Source: CAD feature listing. Evaluate the final solid. Frame: model axes, mm. A direction names the side the tool comes from. Give positions to 0.01 mm unless a question says otherwise; leave off trailing zeros. Order: outer loops, then holes, each group sorted by start corner. A loop starts at its lowest first (then second) coordinate and runs counter-clockwise, first axis right, second up. Notation, with made-up numbers: (58.5, 11.5) - (96.5, 11.5) arc R15 cw to (96.5, 21.5) - close; hole circle Ø6 at (28.5, -14.75). An arc over 180 degrees is marked (long way). Use CSV: the item, a comma, the result in double quotes.
```python
from build123d import *

# Parameters (mm, degrees)
F0_W      = 38.1
F0_H      = 19.05
F1_DEPTH  = 50.8
F3_D      = 9.8044
F4_W      = 50.8
F4_H      = 19.05
F4_H_2    = 38.1
F5_DEPTH  = 12.7
F7_W      = 40.64
F7_H      = 43.18
F8_DEPTH  = 69.85
F9_W      = 40.64
F9_H      = 43.18
F10_DEPTH = 6.35
F12_DEPTH = 9.525
F14_D     = 3.4544
F14_DEPTH = 12.7
F14_TIP   = 1.0378064612
F15_R     = 12.7
F16_R     = 12.7
F17_R     = 4.7625
F19_DEPTH = 25.4


with BuildPart() as f1:
    # F0 (on Right) → F1 (new body)
    with BuildSketch(Plane.YZ):
        Polygon((0, 63.5), (0, 0), (19.05, 0), (57.15, 0), (76.2, 0), (76.2, 63.5), align=None)
        with Locations((38.1, -9.525)):
            Rectangle(F0_W, F0_H)
    extrude(amount=F1_DEPTH)

    # F3 (through all)
    with Locations(Plane(origin=(0, 0, 0), x_dir=(0, -1, 0), z_dir=(-1, 0, 0))):
        with Locations((-38.1, 31.75)):
            Hole(F3_D / 2)

    # F4 (on face) → F5 (join)
    with BuildSketch(Plane(origin=(0, 0, -19.05), x_dir=(1, 0, 0), z_dir=(0, 0, -1))):
        with Locations((25.4, -9.525)):
            Rectangle(F4_W, F4_H)
        with Locations((25.4, -66.675)):
            Rectangle(F4_W, F4_H)
        with Locations((25.4, -38.1)):
            Rectangle(F4_W, F4_H_2)
    extrude(amount=F5_DEPTH)

    # F7 (on face) → F8 (cut)
    with BuildSketch(Plane.XZ):
        with Locations((30.48, 31.75)):
            Rectangle(F7_W, F7_H)
    extrude(amount=-F8_DEPTH, mode=Mode.SUBTRACT)

    # F9 (on face) → F10 (cut)
    with BuildSketch(Plane.XZ):
        with Locations((30.48, 31.75)):
            Rectangle(F9_W, F9_H)
        Polygon((50.8, 53.34), (50.8, 56.515), (6.985, 56.515), (6.985, 6.985), (50.8, 6.985), (50.8, 10.16), (10.16, 10.16), (10.16, 53.34), align=None)
    extrude(amount=-F10_DEPTH, mode=Mode.SUBTRACT)

    # F11 (on face) → F12 (cut)
    with BuildSketch(Plane.YZ.offset(50.8)):
        Polygon((19.05, -19.05), (0, -19.05), (0, -31.75), (76.2, -31.75), (76.2, -19.05), (57.15, -19.05), align=None)
    extrude(amount=-F12_DEPTH, mode=Mode.SUBTRACT)

    # F14
    with Locations(Plane.YZ.offset(50.8)):
        with Locations((12.7, 58.42), (63.5, 58.42), (12.7, 5.08), (63.5, 5.08)):
            Hole(F14_D / 2, depth=F14_DEPTH)
            with Locations((0, 0, -(F14_DEPTH + F14_TIP / 2))):  # 118° drill point
                Cone(0, F14_D / 2, F14_TIP, mode=Mode.SUBTRACT)

    # F15
    f15_edges = [f1.edges().sort_by_distance(p)[0] for p in [
        (30.48, 69.85, 53.34),
    ]]
    fillet(f15_edges, radius=F15_R)

    # F16
    f16_edges = [f1.edges().sort_by_distance(p)[0] for p in [
        (30.48, 69.85, 10.16),
    ]]
    fillet(f16_edges, radius=F16_R)

    # F17
    f17_edges = [f1.edges().sort_by_distance(p)[0] for p in [
        (6.985, 3.175, 56.515),
        (6.985, 3.175, 6.985),
    ]]
    fillet(f17_edges, radius=F17_R)

    # F18 (on face) → F19 (cut)
    with BuildSketch(Plane.XY.offset(63.5)):
        with BuildLine():
            ThreePointArc((25.0825, 15.08125), (26.7662980227, 14.3837980227), (27.46375, 12.7))
            ThreePointArc((27.46375, 12.7), (26.7662980227, 11.0162019773), (25.0825, 10.31875))
            Line((25.0825, 10.31875), (32.7025, 10.31875))
            ThreePointArc((32.7025, 10.31875), (30.32125, 12.7), (32.7025, 15.08125))
            Line((32.7025, 15.08125), (25.0825, 15.08125))
        make_face()
        with BuildLine():
            ThreePointArc((35.08375, 12.7), (34.3862980227, 14.3837980227), (32.7025, 15.08125))
            ThreePointArc((32.7025, 15.08125), (30.32125, 12.7), (32.7025, 10.31875))
            ThreePointArc((32.7025, 10.31875), (34.3862980227, 11.0162019773), (35.08375, 12.7))
        make_face()
        with BuildLine():
            ThreePointArc((25.0825, 10.31875), (26.7662980227, 11.0162019773), (27.46375, 12.7))
            ThreePointArc((27.46375, 12.7), (26.7662980227, 14.3837980227), (25.0825, 15.08125))
            ThreePointArc((25.0825, 15.08125), (22.70125, 12.7), (25.0825, 10.31875))
        make_face()
    extrude(amount=-F19_DEPTH, mode=Mode.SUBTRACT)


solid = f1.part
```
Item 1: Mould query, pull axis Z, two halves, no side actions, for faces 1 (the flat face through (50.8, 50, 7)), 2 (the flat face through (9, 6.35, 34)). Classes: released by +Z, released by -Z, zero draft, split by the parting line, or undercut.
Filled in:
face 1,"zero draft"
face 2,"undercut"
Item 2: First-contact query: pin 1 (11.5 mm diameter, centred on y = 38.1, z = 31.75, fed in from -X); pin 2 (13 mm diameter, centred on y = 42, z = 26.5, fed in from +X); pin 3 (22 mm diameter, centred on x = 21, z = 35.5, fed in from -Y); pin 4 (6.5 mm diameter, centred on y = 34, z = -27.5, fed in from +X) (3 decimals). Flat tips, straight axial feed; report the tip coordinate or a pass-through.
Filled in:
pin 1,"stops at x = 0"
pin 2,"stops at x = 10.16"
pin 3,"stops at y = 6.35"
pin 4,"stops at x = 41.275"
Item 3: Material intervals for line 1 (Y direction, x = 45.5, z = 5.08); line 2 (Z direction, x = 36, y = 15); line 3 (Z direction, x = 42.75, y = 12.7), sorted ascending. Write a range as from..to.
Filled in:
line 1,"y = 0..10.97, 14.43..61.77, 65.23..76.2"
line 2,"z = -31.75..-19.05, 0..10.16, 53.34..63.5"
line 3,"z = 0..3.35, 6.81..10.16, 53.34..56.69, 60.15..63.5"
Item 4: Section D-D on z = 44. Return the cut outline in (x, y) (3 decimals), then the cut area to 3 significant figures.
Filled in:
outline,"(0, 0) - (6.985, 0) - (6.985, 6.35) - (10.16, 6.35) - (10.16, 69.397) - (50.8, 69.397) - (50.8, 76.2) - (0, 76.2) - close"
area,"1,030 mm2"
Item 5: Set-up query: faces 3 (the flat face through (41.275, 38, -25)), 4 (the flat face through (29, 10.319, 58)), 5 (the cylindrical face through (44.361, 63.725, 60.133)), 6 (the flat face through (32, 3, 56.515)). Return all of +Z, -Z, +X, -X, +Y, -Y with unobstructed straight access to the full face (end or side cutting, diameter ignored); none if empty.
Filled in:
face 3,"-Z, +X, +Y, -Y"
face 4,"+Z"
face 5,"+X"
face 6,"+X, -Y"
Item 6: Section B-B on y = 38.1. Return the cut outline in (x, z) (3 decimals).
Filled in:
outline,"(0, -31.75) - (41.275, -31.75) - (41.275, -19.05) - (50.8, -19.05) - (50.8, 10.16) - (10.16, 10.16) - (10.16, 26.848) - (0, 26.848) - close; (0, 36.652) - (10.16, 36.652) - (10.16, 53.34) - (50.8, 53.34) - (50.8, 63.5) - (0, 63.5) - close"
Item 7: Section C-C on x = 24. Return the cut outline in (y, z) (3 decimals), then the cut area to 3 significant figures.
Filled in:
outline,"(0, -31.75) - (76.2, -31.75) - (76.2, -19.05) - (57.15, -19.05) - (57.15, 0) - (76.2, 0) - (76.2, 63.5) - (14.821, 63.5) - (14.821, 53.34) - (57.15, 53.34) arc R12.7 cw to (69.85, 40.64) - (69.85, 22.86) arc R12.7 cw to (57.15, 10.16) - (6.35, 10.16) - (6.35, 6.985) - (0, 6.985) - (0, 0) - (19.05, 0) - (19.05, -19.05) - (0, -19.05) - close; (0, 56.515) - (6.35, 56.515) - (6.35, 53.34) - (10.579, 53.34) - (10.579, 63.5) - (0, 63.5) - close"
area,"3,500 mm2"
Item 8: Section A-A on x = 40. Return the cut outline in (y, z) (3 decimals).
Filled in:
outline,"(0, -31.75) - (76.2, -31.75) - (76.2, -19.05) - (57.15, -19.05) - (57.15, 0) - (76.2, 0) - (76.2, 63.5) - (0, 63.5) - (0, 56.515) - (6.35, 56.515) - (6.35, 53.34) - (57.15, 53.34) arc R12.7 cw to (69.85, 40.64) - (69.85, 22.86) arc R12.7 cw to (57.15, 10.16) - (6.35, 10.16) - (6.35, 6.985) - (0, 6.985) - (0, 0) - (19.05, 0) - (19.05, -19.05) - (0, -19.05) - close; hole circle Ø3.454 at (12.7, 5.08); hole circle Ø3.454 at (12.7, 58.42); hole circle Ø3.454 at (63.5, 5.08); hole circle Ø3.454 at (63.5, 58.42)"
